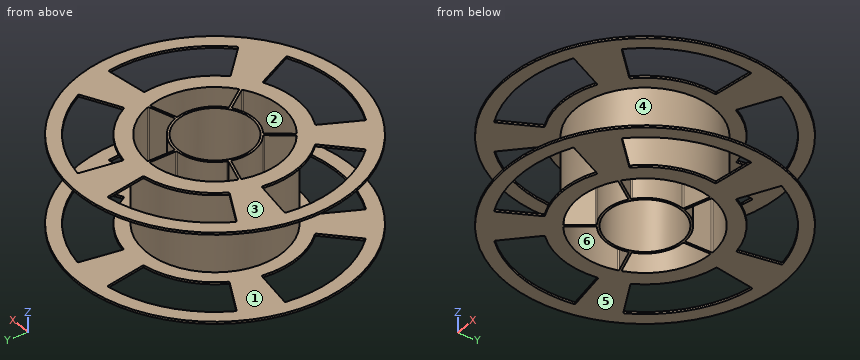
```python
from build123d import *

# Parameters (mm, degrees)
POCKET002_DEPTH    = 646.737672396
POLARPATTERN_COUNT = 5


with BuildPart() as part:
    # Sketch010 → Revolution001 (revolve)
    with BuildSketch(Plane.XZ):
        Polygon((26.75, 32.95), (26.75, -32.95), (100, -32.95), (100, -31.35), (49.75, -31.35), (49.75, 31.35), (100, 31.35), (100, 32.95), align=None)
    revolve(axis=Axis((0, 0, 0), (0, 0, 1)))

    # Sketch012 (on Face8 of Revolution001) → Pocket002 (cut, through all)
    with BuildSketch(Plane(origin=(0, 0, 32.95), x_dir=(-1, 0, 0), z_dir=(0, 0, 1))):
        with BuildLine():
            ThreePointArc((15.3796885804, 23.8157023657), (0, 28.35), (-15.3796885804, 23.8157023657))
            ThreePointArc((-16.4608969153, 24.0175222024), (-15.9604769906, 23.7013334549), (-15.3796885804, 23.8157023657))
            Line((-16.4608969153, 24.0175222024), (-27.1685241193, 38.755306697))
            ThreePointArc((-26.9694002475, 39.888268329), (-27.3092336515, 39.3640164673), (-27.1685241193, 38.755306697))
            ThreePointArc((26.9694002475, 39.888268329), (0, 48.15), (-26.9694002475, 39.888268329))
            ThreePointArc((27.1685241193, 38.755306697), (27.3092336515, 39.3640164673), (26.9694002475, 39.888268329))
            Line((16.4608969153, 24.0175222024), (27.1685241193, 38.755306697))
            ThreePointArc((15.3796885804, 23.8157023657), (15.9604769906, 23.7013334549), (16.4608969153, 24.0175222024))
        make_face()
        with BuildLine():
            ThreePointArc((25.9449786764, 53.823048794), (0, 59.75), (-25.9449786764, 53.823048794))
            ThreePointArc((-27.0083499061, 54.1868206795), (-26.5513009975, 53.7867581012), (-25.9449786764, 53.823048794))
            Line((-27.0083499061, 54.1868206795), (-39.7895658353, 79.8297591794))
            ThreePointArc((-39.4240107242, 80.9057932315), (-39.8310568512, 80.4439657297), (-39.7895658353, 79.8297591794))
            ThreePointArc((39.4240107242, 80.9057932315), (0, 90), (-39.4240107242, 80.9057932315))
            ThreePointArc((39.7895658353, 79.8297591794), (39.8310568512, 80.4439657297), (39.4240107242, 80.9057932315))
            Line((27.0083499061, 54.1868206795), (39.7895658353, 79.8297591794))
            ThreePointArc((25.9449786764, 53.823048794), (26.5513009975, 53.7867581012), (27.0083499061, 54.1868206795))
        make_face()
    pocket002 = extrude(amount=-POCKET002_DEPTH, mode=Mode.SUBTRACT)

    # PolarPattern: Pocket002 ×5 about axis
    polarpattern_axis = Axis((0, 0, 32.95), (0, 0, 1))
    for i in range(1, POLARPATTERN_COUNT):
        add(pocket002.rotate(polarpattern_axis, i * 360 / POLARPATTERN_COUNT), mode=Mode.SUBTRACT)


solid = part.part
```
Geometry check sheet. Reference: the model listing, model coordinates, mm. Face numbers are marked on the shaded views. A direction names the side the tool comes from. Round coordinates to 2 decimals unless told otherwise and drop trailing zeros. Loops run counter-clockwise (first coordinate to the right, second up) from the corner with the lowest first, then second, coordinate; pieces in that order, holes last. Notation, with made-up numbers: M 87.5,10 L 135.5,10 A29 ccw 135.5,48 Z; hole C -0.5,49 d1. An arc over 180 degrees is marked long. Return JSON: item names as keys, results as strings. Group by question number.
(1) Mould release check, pull along Z, two halves, no side actions. Record for the marked faces 3, 4, 5 and 6: pulls with the +Z half, pulls with the -Z half, needs draft (parallel to the pull), parting line crosses it, or undercut.
(2) Section check A-A, the plane y = -67.5. Enter the section's corners in (x, z), and give its area (3 significant figures).
(3) Go/stop test with flat-tipped pins: pin 1 (5 mm diameter, centred on y = 44, z = 19, fed in from -X); pin 2 (12 mm diameter, centred on y = 47, z = 20, fed in from -X); pin 3 (2 mm diameter, centred on x = -12.5, z = 0, fed in from -Y). Record where each tip stops, or that it passes through.
(4) Section check B-B, the plane x = -82. Enter the section's corners in (y, z), and give its area (3 significant figures).
(5) Section check C-C, the plane y = 0. Give the number of separate pieces and of enclosed holes in the cut face, and give its area (3 significant figures).
(6) Scan lines: line 1 along Y through (x, z) = (0, 1); line 2 along Z through (x, y) = (-31, -54.5); line 3 along Y through (x, z) = (11, -26.5). Record each from-to range of solid material in increasing order. Write a range as [from, to].
(7) Set-up check for the marked faces 1 and 2: record each of +Z, -Z, +X, -X, +Y, -Y from which the full face is reachable in a straight line by a thin tool's end or side.
Data:
{
 "1": {"face 3": "pulls with the +Z half", "face 4": "undercut", "face 5": "pulls with the -Z half", "face 6": "needs draft"},
 "2": {"outline": "M -73.78,-32.95 L -33.64,-32.95 L -33.64,-31.35 L -73.78,-31.35 Z; M -73.78,31.35 L -33.64,31.35 L -33.64,32.95 L -73.78,32.95 Z; M 33.64,-32.95 L 73.78,-32.95 L 73.78,-31.35 L 33.64,-31.35 Z; M 33.64,31.35 L 73.78,31.35 L 73.78,32.95 L 33.64,32.95 Z", "area": "257 mm²"},
 "3": {"pin 1": "x = -27.44", "pin 2": "x = -28.18", "pin 3": "y = -48.4"},
 "4": {"outline": "M -57.24,-32.95 L -37.09,-32.95 L -37.09,-31.35 L -57.24,-31.35 Z; M -57.24,31.35 L -37.09,31.35 L -37.09,32.95 L -57.24,32.95 Z; M 12.24,-32.95 L 57.24,-32.95 L 57.24,-31.35 L 12.24,-31.35 Z; M 12.24,31.35 L 57.24,31.35 L 57.24,32.95 L 12.24,32.95 Z", "area": "208 mm²"},
 "5": {"separate pieces": "8", "enclosed holes": "0", "area": "550 mm²"},
 "6": {"line 1": "[-49.75, -48.15], [-28.35, -26.75], [26.75, 49.75]", "line 2": "[-32.95, -31.35], [31.35, 32.95]", "line 3": "[-48.52, -46.88], [-26.13, -24.38], [24.38, 26.13], [46.88, 48.52]"},
 "7": {"face 1": "none", "face 2": "+Z, -Z"}
}
